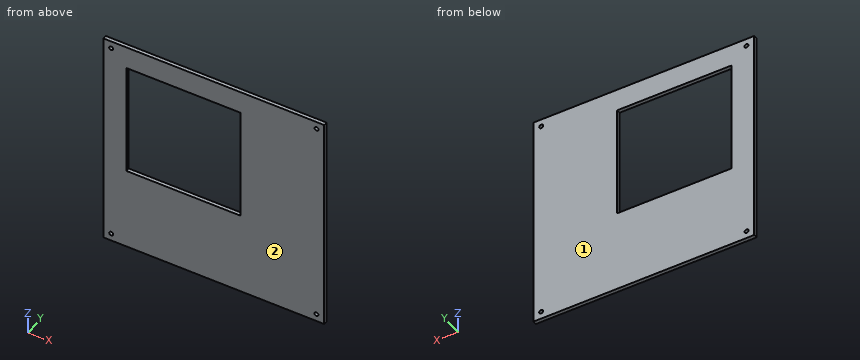
from build123d import *

# Parameters (mm, degrees)
F0_W     = 290
F0_H     = 290
F1_DEPTH = 5
F2_R     = 2.6
F3_DEPTH = 5.001
F4_W     = 150
F4_H     = 150
F5_DEPTH = 5.001


with BuildPart() as f1:
    # F0 (on Front) → F1 (new body)
    with BuildSketch(Plane.XZ):
        Rectangle(F0_W, F0_H)
    extrude(amount=F1_DEPTH)

    # F2 (on face) → F3 (cut, through all)
    with BuildSketch(Plane.XZ.offset(5)):
        with Locations((-135, 135)):
            Circle(F2_R)
        with Locations((-135, -135)):
            Circle(F2_R)
        with Locations((135, 135)):
            Circle(F2_R)
        with Locations((135, -135)):
            Circle(F2_R)
        with Locations((405, 135)):
            Circle(F2_R)
        with Locations((405, -135)):
            Circle(F2_R)
    extrude(amount=-F3_DEPTH, mode=Mode.SUBTRACT)

    # F4 (on face) → F5 (cut, through all)
    with BuildSketch(Plane.XZ.offset(5)):
        with Locations((-40, 40)):
            Rectangle(F4_W, F4_H)
    extrude(amount=-F5_DEPTH, mode=Mode.SUBTRACT)


solid = f1.part
The listing builds one solid part. Answer for the finished solid, in the listing's coordinates (mm). Face numbers are marked on the shaded views. Give positions to 0.01 mm unless a question says otherwise; leave off trailing zeros. Write each loop counter-clockwise with the first axis right and the second up, starting at its lowest first coordinate (ties: lowest second). Pieces come first, ordered by that corner, then holes. Notation, with made-up numbers: (0, 45) - (5, 45) arc R25 ccw to (5, 70) - close; hole circle Ø1 at (9.25, 13.25). An arc over 180 degrees is marked (long way). Use a Markdown table: item, result.
1. Section A-A on z = -21.5 is taken. Write down the section's boundary in (x, y).
Values follow:
| item | result |
|---|---|
| outline | (-145, -5) - (-115, -5) - (-115, 0) - (-145, 0) - close; (35, -5) - (145, -5) - (145, 0) - (35, 0) - close |
2. Section C-C on y = -1.6 is taken. Write down the section's boundary in (x, z).
Values follow:
| item | result |
|---|---|
| outline | (-145, -145) - (145, -145) - (145, 145) - (-145, 145) - close; hole circle Ø5.2 at (-135, -135); hole circle Ø5.2 at (-135, 135); hole (-115, -35) - (35, -35) - (35, 115) - (-115, 115) - close; hole circle Ø5.2 at (135, -135); hole circle Ø5.2 at (135, 135) |
3. Each of these flat-tipped pins is pushed along its axis until it touches: P1, Ø4.5, axis at x = -135, z = -135, coming from the +Y side; P2, Ø3, axis at x = 35, z = -82, coming from the +Y side. Where does it stop, or does it pass through?
Values follow:
| item | result |
|---|---|
| P1 | passes through |
| P2 | stops at y = 0 |
4. Find the intervals of material crossed by probe 1 along X at (y, z) = (-3.45, -135); probe 2 along X at (y, z) = (-1.25, 21); probe 3 along Z at (x, y) = (-74, -1.7), in increasing order. Write a range as from..to.
Values follow:
| item | result |
|---|---|
| probe 1 | x = -145..-137.6, -132.4..132.4, 137.6..145 |
| probe 2 | x = -145..-115, 35..145 |
| probe 3 | z = -145..-35, 115..145 |
5. For a pull along Y with two mould halves and no side action, classify the marked faces 1 and 2 as released by +Y, released by -Y, zero draft, split by the parting line, or undercut.
Values follow:
| item | result |
|---|---|
| face 1 | released by +Y |
| face 2 | released by -Y |
6. Section B-B on x = -64 is taken. Write down the section's boundary in (y, z), plus the area to 3 significant figures.
Values follow:
| item | result |
|---|---|
| outline | (-5, -145) - (0, -145) - (0, -35) - (-5, -35) - close; (-5, 115) - (0, 115) - (0, 145) - (-5, 145) - close |
| area | 700 mm² |
